Autodesk Inventor part; units mm, degrees
ref_plane "YZ Plane" through (0, 0, 0) normal (1, 0, 0) x (0, 1, 0)
ref_plane "XZ Plane" through (0, 0, 0) normal (0, 1, 0) x (-1, 0, 0)
ref_plane "XY Plane" through (0, 0, 0) normal (0, 0, 1) x (1, 0, 0)
sketch "스케치1" plane through (0, 0, 0) normal (0, 1, 0) x (-1, 0, 0)
  line L0 (-8, 15.75) -> (8, 15.75)
  line L1 (8, 15.75) -> (8, -15.75)
  line L2 (8, -15.75) -> (-8, -15.75)
  line L3 (-8, -15.75) -> (-8, 15.75)
  line L4 (-8, 15.75) -> (8, -15.75) construction
  line L5 (8, 15.75) -> (-8, -15.75) construction
  point P0 (0, 0)
  dimension "d0" = 16
  dimension "d1" = 31.5
extrude "돌출1" add sketch "스케치1" along normal blind 13.5
sketch "스케치2" plane through (0, 13.5, 0) normal (0, 1, 0) x (1, 0, 0)
  line L0 (-8, -21.5) -> (8, -21.5)
  line L1 (8, -21.5) -> (8, 21.5)
  line L2 (8, 21.5) -> (-8, 21.5)
  line L3 (-8, 21.5) -> (-8, -21.5)
  line L4 (-8, -21.5) -> (8, 21.5) construction
  line L5 (8, -21.5) -> (-8, 21.5) construction
  circle A0 centre (-4.25, -18.5) radius 2
  line L6 (0, 0) -> (0, -2.2737)
  line L7 (0, 0) -> (-1.7913, 0)
  circle A1 centre (4.25, -18.5) radius 2
  circle A2 centre (-4.25, 18.5) radius 2
  circle A3 centre (4.25, 18.5) radius 2
  point P0 (-8, 15.75)
  dimension "d4" = 43
  dimension "d5" = 4
  dimension "d6" = 37
  dimension "d7" = 8.5
extrude "돌출2" add sketch "스케치2" along normal blind 2.3
extrude "돌출3" add sketch "스케치1" along normal blind 22.2
sketch "스케치4" plane through (0, 22.2, 0) normal (0, 1, 0) x (1, 0, 0)
  circle A0 centre (0, 7.75) radius 2.75
  line L0 (8, 15.75) -> (-8, 15.75)
  line L1 (-1.5811, 10) -> (1.5811, 10)
  point P0 (0, 0)
  dimension "d12" = 8
  dimension "d13" = 5.5
  dimension "d14" = 0.5
extrude "돌출4" add sketch "스케치4" along normal blind 4.5 contours A0 L1 picked at (-0.1073, 8.3396)
properties part number "감속기어 모터'"
Can you work these out from the model? Positions are in its coordinate system, mm. A direction names the side the tool comes from. Round coordinates to 2 decimals unless told otherwise and drop trailing zeros. Write each loop counter-clockwise with the first axis right and the second up, starting at its lowest first coordinate (ties: lowest second). Pieces come first, ordered by that corner, then holes. Notation, with made-up numbers: (-22.75, 28.5) -> (17.25, 28.5) arc R8 cw to (17.25, 40.5) -> close; hole circle Ø8 at (-22.75, 81.5). An arc over 180 degrees is marked (long way). Use one line per item in the form item = value. Start each with the question number.
Q1. Imagine slicing it at A-A (y = 14.25). Please give me the cut outline in (x, z), then the cut area to 3 significant figures.
Q2. I'm going to push flat-ended pins straight in: P1, Ø7, axis at x = 3, y = 8, coming from the +Z side; P2, Ø3.5, axis at x = 0.5, y = 24, coming from the -Z side; P3, Ø2, axis at y = 13, z = 16, coming from the -X side; P4, Ø5, axis at x = 2.5, y = 20, coming from the -Z side. Where does each tip first touch, or does it pass through?
Q3. Imagine slicing it at B-B (z = 18.5). Please give me the cut outline in (x, y).
Q4. We'd pull the mould along X, two halves only. Please class faces 1 (the face through (0, 24, -10)), 2 (the face through (8, 11, 0)), 3 (the face through (-4.51, 14.634, -16.517)), 4 (the face through (3.99, 14.634, 20.483)): +X half, -X half, draft (parallel to the pull), parting line (faces both ways), or undercut.
Q5. Which directions (+Z, -Z, +X, -X, +Y, -Y) give clear straight access to the entire face, cutting with the end or side of a thin tool? Please do faces 5 (the face through (0, 15.8, 19)), 6 (the face through (0, 13.5, -19)), 7 (the face through (0, 19, -15.75)).
Q6. Imagine slicing it at C-C (x = 0). Please give me the cut outline in (y, z), then the cut area to 3 significant figures.
Q7. Imagine slicing it at D-D (x = 4.25). Please give me the cut outline in (y, z), then the cut area to 3 significant figures.
Q8. If I drill on probe 1 along X at (y, z) = (14.75, -18.5); probe 2 along Z at (x, y) = (4.25, 15.15); probe 3 along Z at (x, y) = (3.75, 15.25), over which ranges is the centre line in solid material (lowest first)? Write a range as [from, to].
Worked out:
q1.outline = (-8, -21.5) -> (8, -21.5) -> (8, 21.5) -> (-8, 21.5) -> close; hole circle Ø4 at (-4.25, -18.5); hole circle Ø4 at (-4.25, 18.5); hole circle Ø4 at (4.25, -18.5); hole circle Ø4 at (4.25, 18.5)
q1.area = 638 mm^2
q2.P1 = 15.75
q2.P2 = -10
q2.P3 = -8
q2.P4 = -15.75
q3.outline = (-8, 13.5) -> (-6.25, 13.5) -> (-6.25, 15.8) -> (-8, 15.8) -> close; (-2.25, 13.5) -> (2.25, 13.5) -> (2.25, 15.8) -> (-2.25, 15.8) -> close; (6.25, 13.5) -> (8, 13.5) -> (8, 15.8) -> (6.25, 15.8) -> close
q4.face_1 = draft
q4.face_2 = +X half
q4.face_3 = undercut
q4.face_4 = undercut
q5.face_5 = +Z, +X, -X, +Y
q5.face_6 = -Z, +X, -X, -Y
q5.face_7 = -Z, +X, -X, +Y
q6.outline = (0, -15.75) -> (13.5, -15.75) -> (13.5, -21.5) -> (15.8, -21.5) -> (15.8, -15.75) -> (22.2, -15.75) -> (22.2, -10) -> (26.7, -10) -> (26.7, -5) -> (22.2, -5) -> (22.2, 15.75) -> (15.8, 15.75) -> (15.8, 21.5) -> (13.5, 21.5) -> (13.5, 15.75) -> (0, 15.75) -> close
q6.area = 748 mm^2
q7.outline = (0, -15.75) -> (13.5, -15.75) -> (13.5, -16.5) -> (15.8, -16.5) -> (15.8, -15.75) -> (22.2, -15.75) -> (22.2, 15.75) -> (15.8, 15.75) -> (15.8, 16.5) -> (13.5, 16.5) -> (13.5, 15.75) -> (0, 15.75) -> close; (13.5, -21.5) -> (15.8, -21.5) -> (15.8, -20.5) -> (13.5, -20.5) -> close; (13.5, 20.5) -> (15.8, 20.5) -> (15.8, 21.5) -> (13.5, 21.5) -> close
q7.area = 707 mm^2
q8.probe_1 = [-8, -6.25], [-2.25, 2.25], [6.25, 8]
q8.probe_2 = [-21.5, -20.5], [-16.5, 16.5], [20.5, 21.5]
q8.probe_3 = [-21.5, -20.44], [-16.56, 16.56], [20.44, 21.5]
